Check sheet for the modelled part. Datum: model origin and axes. Units: mm. A direction names the side the tool comes from. Round coordinates to 2 decimals unless told otherwise and drop trailing zeros. Order: outer loops, then holes, each group sorted by start corner. A loop starts at its lowest first (then second) coordinate and runs counter-clockwise, first axis right, second up. Notation, with made-up numbers: (27, 37) -> (74, 37) arc R16 cw to (74, 66) -> close; hole circle Ø2 at (-6, 58.25). An arc over 180 degrees is marked (long way). Answer in a Markdown table with one row per item.
from build123d import *

# Parameters (mm, degrees)
SKETCH2_R           = 57.15
BOSS_EXTRUDE1_DEPTH = 9.525


with BuildPart() as part:
    # Sketch1 → Revolve1 (revolve)
    with BuildSketch(Plane.XY):
        Polygon((-30.1625, -57.15), (30.1625, -57.15), (30.1625, 0), (20.6375, 0), (20.6375, -51.1302), (-30.1625, -51.1302), align=None)
    revolve(axis=Axis((-30.1625, 0, 0), (1, 0, 0)))

    # Sketch2 → Boss-Extrude1 (add)
    with BuildSketch(Plane(origin=(30.1625, 0, 0), x_dir=(0, 0, -1), z_dir=(1, 0, 0))):
        Polygon((0, 66.907679321), (-57.94375, 33.45383966), (-57.94375, -33.45383966), (0, -66.907679321), (57.94375, -33.45383966), (57.94375, 33.45383966), align=None)
        Circle(SKETCH2_R, mode=Mode.SUBTRACT)
    extrude(amount=-BOSS_EXTRUDE1_DEPTH)


solid = part.part
Item 1: Set-up check for faces 4 (the flat face through (30.162, 1, 1)), 5 (the flat face through (20.638, -49, 30)): record each of +Z, -Z, +X, -X, +Y, -Y from which the full face is reachable in a straight line by a thin tool's end or side.
Result sheet:
| item | result |
|---|---|
| face 4 | +Z, -Z, +X, +Y, -Y |
| face 5 | -X |
Item 2: Cross-section at B-B (x = 14). Record the boundary of the cut face in (y, z).
Result sheet:
| item | result |
|---|---|
| outline | circle Ø114.3 at (0, 0); hole circle Ø102.26 at (0, 0) |
Item 3: Mould release check, pull along Z, two halves, no side actions. Record for faces 1 (the flat face through (25, 0, 57.944)), 2 (the flat face through (20.637, -1, -1)), 3 (the cylindrical face through (-4.4, -54.5, -17.2)): pulls with the +Z half, pulls with the -Z half, needs draft (parallel to the pull), parting line crosses it, or undercut.
Result sheet:
| item | result |
|---|---|
| face 1 | pulls with the +Z half |
| face 2 | undercut |
| face 3 | parting line crosses it |
Item 4: Scan lines: line 1 (Z direction, x = 2, y = 0); line 2 (X direction, y = 34.5, z = -13). Record each from-to range of solid material in increasing order. Write a range as [from, to].
Result sheet:
| item | result |
|---|---|
| line 1 | z = [-57.15, -51.13], [51.13, 57.15] |
| line 2 | x = [20.64, 30.16] |
Item 5: Cross-section at A-A (y = 0). Record the boundary of the cut face in (x, z), and give its area (3 significant figures).
Result sheet:
| item | result |
|---|---|
| outline | (-30.16, -57.15) -> (20.64, -57.15) -> (20.64, -57.94) -> (30.16, -57.94) -> (30.16, 57.94) -> (20.64, 57.94) -> (20.64, 57.15) -> (-30.16, 57.15) -> (-30.16, 51.13) -> (20.64, 51.13) -> (20.64, -51.13) -> (-30.16, -51.13) -> close |
| area | 1,720 mm^2 |
Item 6: Cross-section at C-C (z = -8.5). Record the boundary of the cut face in (x, y).
Result sheet:
| item | result |
|---|---|
| outline | (-30.16, -56.51) -> (20.64, -56.51) -> (20.64, -62) -> (30.16, -62) -> (30.16, 62) -> (20.64, 62) -> (20.64, 56.51) -> (-30.16, 56.51) -> (-30.16, 50.42) -> (20.64, 50.42) -> (20.64, -50.42) -> (-30.16, -50.42) -> close |
Item 7: Depth check by flat-ended pin: P1, Ø5, axis at x = -18, z = -42, coming from the -Y side; P2, Ø10, axis at x = -16, z = -46, coming from the -Y side; P3, Ø5, axis at x = -24, y = 8.5, coming from the -Z side. Enter the tip coordinate at first touch or a pass-through.
Result sheet:
| item | result |
|---|---|
| P1 | stops at y = -41.3 |
| P2 | stops at y = -39.81 |
| P3 | stops at z = -56.83 |
